Design review of the part built by this model. Coordinates are the model's own, in mm. Give positions to 0.01 mm unless a question says otherwise; leave off trailing zeros. Order: outer loops, then holes, each group sorted by start corner. A loop starts at its lowest first (then second) coordinate and runs counter-clockwise, first axis right, second up. Notation, with made-up numbers: (-4.75, -19) -> (26.25, -19) arc R20 ccw to (26.25, 15) -> close; hole circle Ø9 at (-17, 29). An arc over 180 degrees is marked (long way). Return JSON: item names as keys, results as strings.
Autodesk Inventor part; units mm, degrees
ref_plane "YZ Plane" through (0, 0, 0) normal (1, 0, 0) x (0, 1, 0)
ref_plane "XZ Plane" through (0, 0, 0) normal (0, 1, 0) x (-1, 0, 0)
ref_plane "XY Plane" through (0, 0, 0) normal (0, 0, 1) x (1, 0, 0)
sketch "Sketch1" plane through (0, 0, 0) normal (1, 0, 0) x (0, 1, 0)
  line L0 (-31.5, 71.75) -> (31.5, 71.75)
  line L1 (31.5, 71.75) -> (31.5, -71.75)
  line L2 (31.5, -71.75) -> (-31.5, -71.75)
  line L3 (-31.5, -71.75) -> (-31.5, 71.75)
  line L4 (-31.5, 71.75) -> (31.5, -71.75) construction
  line L5 (31.5, 71.75) -> (-31.5, -71.75) construction
  line L6 (12.4, 71.75) -> (24.4, 71.75)
  line L7 (6.3, 71.75) -> (15.5, 71.75)
  line L8 (15.5, 71.75) -> (15.5, 66.75)
  line L9 (15.5, 66.75) -> (6.3, 66.75)
  line L10 (6.3, 66.75) -> (6.3, 71.75)
  line L11 (6.3, 71.75) -> (15.5, 66.75) construction
  line L12 (15.5, 71.75) -> (6.3, 66.75) construction
  line L13 (22.3, 66.75) -> (31.5, 66.75)
  line L14 (31.5, 66.75) -> (31.5, 71.75)
  line L15 (31.5, 71.75) -> (22.3, 71.75)
  line L16 (22.3, 71.75) -> (22.3, 66.75)
  line L17 (22.3, 66.75) -> (31.5, 71.75) construction
  line L18 (31.5, 66.75) -> (22.3, 71.75) construction
  line L19 (-9.7, 71.75) -> (-0.5, 71.75)
  line L20 (-0.5, 71.75) -> (-0.5, 66.75)
  line L21 (-0.5, 66.75) -> (-9.7, 66.75)
  line L22 (-9.7, 66.75) -> (-9.7, 71.75)
  line L23 (-9.7, 71.75) -> (-0.5, 66.75) construction
  line L24 (-0.5, 71.75) -> (-9.7, 66.75) construction
  point P0 (0, 0)
  point P1 (10.9, 69.25)
  point P2 (26.9, 69.25)
  point P3 (31.5, 69.25)
  point P4 (22.3, 71.75)
  point P5 (-5.1, 69.25)
  point P6 (-0.5, 71.75)
  dimension "d0" = 143.5
  dimension "d1" = 63
  dimension "d19" = 5
  dimension "d20" = 9.2
  dimension "d21" = 9.2
  dimension "d22" = 5
  dimension "d23" = 16
  dimension "d26" = 6.8
  dimension "d27" = 16
  dimension "d28" = 9.2
extrude "Extrusion1" add sketch "Sketch1" along normal blind 5
extrude "Extrusion3" cut sketch "Sketch1" along normal through all contours L0 L20 L21 L22 | L0 L8 L9 L10 | L13 L16 L0 L1
mirror "Mirror1" about plane through (0, 0, 0) normal (0, 0, 1) of "Extrusion3"
equation "\"d21\" = d20"
equation "\"d22\" = d19"
equation "\"d28\" = d21"
properties part number "gate"
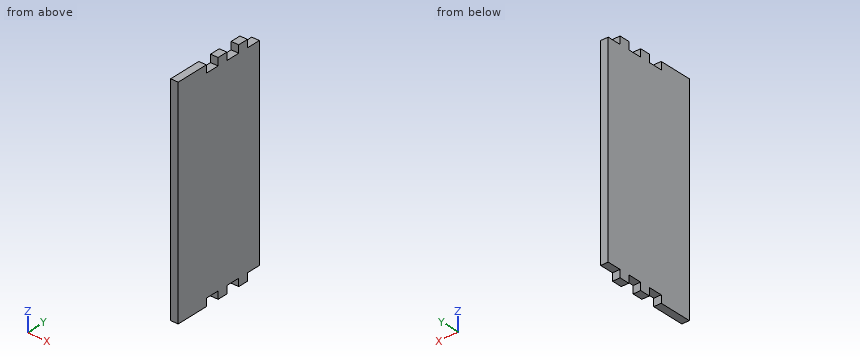
Item 1: For pin 1 (1.5 mm diameter, centred on x = 2.5, z = 69, fed in from +Y); pin 2 (1 mm diameter, centred on y = 2, z = -6.5, fed in from -X); pin 3 (2.5 mm diameter, centred on x = 1.5, y = 12, fed in from +Z), all flat-tipped, find the tip position at first contact; note any pin that passes through.
Result set:
{"pin 1": "stops at y = 22.3", "pin 2": "stops at x = 0", "pin 3": "stops at z = 66.75"}
Item 2: Add section B-B (y = -3). Give the boundary of the cut face in (x, z).
Result set:
{"outline": "(0, -66.75) -> (5, -66.75) -> (5, 66.75) -> (0, 66.75) -> close"}
Item 3: Wall thickness on L1, parallel to Z at x = 1.45, y = -5: over which ranges is the line inside the solid? List them lowest first. Write a range as [from, to].
Result set:
{"L1": "z = [-66.75, 66.75]"}
Item 4: Add section A-A (x = 2.95). Give the boundary of the cut face in (y, z).
Result set:
{"outline": "(-31.5, -71.75) -> (-9.7, -71.75) -> (-9.7, -66.75) -> (-0.5, -66.75) -> (-0.5, -71.75) -> (6.3, -71.75) -> (6.3, -66.75) -> (15.5, -66.75) -> (15.5, -71.75) -> (22.3, -71.75) -> (22.3, -66.75) -> (31.5, -66.75) -> (31.5, 66.75) -> (22.3, 66.75) -> (22.3, 71.75) -> (15.5, 71.75) -> (15.5, 66.75) -> (6.3, 66.75) -> (6.3, 71.75) -> (-0.5, 71.75) -> (-0.5, 66.75) -> (-9.7, 66.75) -> (-9.7, 71.75) -> (-31.5, 71.75) -> close"}
